Design review of the part shown in the three views and the two pictorial views. Dimensions are in mm from the part's minimum x, y and z. Coordinates: 2 decimals unless noted, no trailing zeros. Loops run counter-clockwise (first coordinate to the right, second up) from the corner with the lowest first, then second, coordinate; pieces in that order, holes last. Notation, with made-up numbers: (60, -10.5) - (111, -10.5) arc R13 ccw to (111, 0.5) - close; hole circle Ø2 at (73, -35). An arc over 180 degrees is marked (long way). One line per item, written item: value. Start each with the question number.
1. Take a section at C-C, the plane x = 15.5. State the section outline as (y, z) points.
2. Take a section at B-B, the plane x = 9. Count the separate pieces of the cut face and the enclosed holes in it, and give its area (3 significant figures).
3. Insertion check: pin 1 (1.5 mm diameter, centred on x = 3, y = 54.5, fed in from +Z); pin 2 (4 mm diameter, centred on x = 3.5, y = 57, fed in from -Z); pin 3 (1 mm diameter, centred on x = 4, y = 15.5, fed in from -Z). Each pin has a flat end and moves straight along its axis. Give the tip position at first contact, or say it passes through.
4. The part is to be moulded in two halves that separate along Z. For the marked faces 1 and 2, say which applies: released by +Z, released by -Z, zero draft, split by the parting line, or undercut.
5. Take a section at D-D, the plane y = 88. State the section outline as (x, z) points, and give its area (3 significant figures).
6. To check wall thickness, follow line 1 (Y direction, x = 9, z = 0.2); line 2 (Z direction, x = 9, y = 84.5); line 3 (Z direction, x = 10.75, y = 83). State the ranges of each line that lie inside material, in increasing order. Write a range as from..to.
7. Take a section at A-A, the plane z = 5.25. State the section outline as (x, y) points.
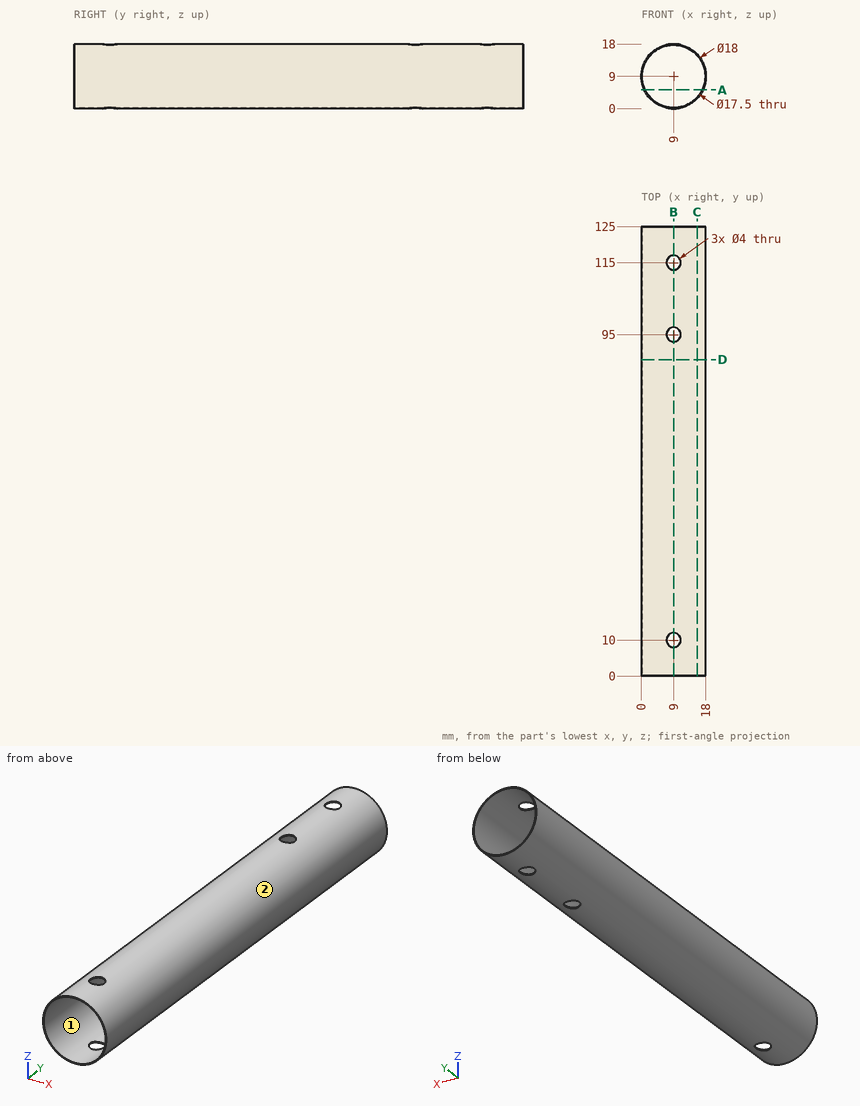
Solutions:
1. outline: (0, 2.78) - (125, 2.78) - (125, 3.14) - (0, 3.14) - close; (0, 14.86) - (125, 14.86) - (125, 15.22) - (0, 15.22) - close
2. separate pieces: 8
2. enclosed holes: 0
2. area: 56.5 mm2
3. pin 1: z = 16.31
3. pin 2: z = 0.71
3. pin 3: z = 1.21
4. face 1: undercut
4. face 2: split by the parting line
5. outline: circle Ø18 at (9, 9); hole circle Ø17.5 at (9, 9)
5. area: 13.9 mm2
6. line 1: 0..8, 12..93, 97..113, 117..125
6. line 2: 0..0.25, 17.75..18
6. line 3: 0.17..0.43, 17.57..17.83
7. outline: (0.82, 0) - (1.09, 0) - (1.09, 125) - (0.82, 125) - close; (16.91, 0) - (17.18, 0) - (17.18, 125) - (16.91, 125) - close
